```python
from build123d import *

# Parameters (mm, degrees)
F0_R     = 1.5875
F0_W     = 3.175
F0_H     = 10.004552
F1_DEPTH = 3.175


# Not quite as in the source:
# - a length typed as a fraction of an inch, garbled in the dataset ("3 / 203.2 mm" for 3/8 in), is restored
# - a feature names something its author has since deleted; it is built from what else it names


with BuildPart() as f1:
    # F0 (on Top) → F1 (new body)
    with BuildSketch(Plane.XY):
        with BuildLine():
            Line((-226.9615088272, -74.910188), (-188.8615088272, -74.910188))
            ThreePointArc((-188.8615088272, -74.910188), (-180.8069453098, -55.4647515174), (-161.3615088272, -47.410188))
            ThreePointArc((-161.3615088272, -47.410188), (-141.9160723446, -55.4647515174), (-133.8615088272, -74.910188))
            Line((-133.8615088272, -74.910188), (-95.7615088272, -74.910188))
            Line((-95.7615088272, -74.910188), (-95.7615088272, 102.889812))
            Line((-95.7615088272, 102.889812), (-226.9615088272, 102.889812))
            Line((-226.9615088272, 102.889812), (-226.9615088272, -74.910188))
        make_face()
        Polygon((-221.8815088272, 50.02276), (-221.8815088272, 60.027312), (-218.7065088272, 60.027312), (-218.7065088272, 50.02276), (-218.7065088272, 40.018208), (-218.7065088272, 30.013656), (-218.7065088272, 20.009104), (-218.7065088272, 10.004552), (-218.7065088272, 0), (-218.7065088272, -10.004552), (-218.7065088272, -20.009104), (-218.7065088272, -30.013656), (-218.7065088272, -40.018208), (-218.7065088272, -50.02276), (-221.8815088272, -50.02276), (-221.8815088272, -40.018208), (-221.8815088272, -30.013656), (-221.8815088272, -20.009104), (-221.8815088272, -10.004552), (-221.8815088272, 0), (-221.8815088272, 10.004552), (-221.8815088272, 20.009104), (-221.8815088272, 30.013656), (-221.8815088272, 40.018208), align=None, mode=Mode.SUBTRACT)
        Polygon((-199.6565088272, 60.027312), (-196.4815088272, 60.027312), (-196.4815088272, 50.02276), (-196.4815088272, 40.018208), (-196.4815088272, 30.013656), (-196.4815088272, 20.009104), (-196.4815088272, 10.004552), (-196.4815088272, 0), (-196.4815088272, -10.004552), (-196.4815088272, -20.009104), (-196.4815088272, -30.013656), (-196.4815088272, -40.018208), (-196.4815088272, -50.02276), (-199.6565088272, -50.02276), (-199.6565088272, -40.018208), (-199.6565088272, -30.013656), (-199.6565088272, -20.009104), (-199.6565088272, -10.004552), (-199.6565088272, 0), (-199.6565088272, 10.004552), (-199.6565088272, 20.009104), (-199.6565088272, 30.013656), (-199.6565088272, 40.018208), (-199.6565088272, 50.02276), align=None, mode=Mode.SUBTRACT)
        with Locations((-186.3334280729, -16.5444072336)):
            Circle(F0_R, mode=Mode.SUBTRACT)
        Polygon((-126.2415088272, 60.027312), (-123.0665088272, 60.027312), (-123.0665088272, 50.02276), (-123.0665088272, 40.018208), (-123.0665088272, 30.013656), (-123.0665088272, 20.009104), (-123.0665088272, 10.004552), (-123.0665088272, 0), (-123.0665088272, -10.004552), (-123.0665088272, -20.009104), (-123.0665088272, -30.013656), (-123.0665088272, -40.018208), (-123.0665088272, -50.02276), (-126.2415088272, -50.02276), (-126.2415088272, -40.018208), (-126.2415088272, -30.013656), (-126.2415088272, -20.009104), (-126.2415088272, -10.004552), (-126.2415088272, 0), (-126.2415088272, 10.004552), (-126.2415088272, 20.009104), (-126.2415088272, 30.013656), (-126.2415088272, 40.018208), (-126.2415088272, 50.02276), align=None, mode=Mode.SUBTRACT)
        Polygon((-104.0165088272, 50.02276), (-104.0165088272, 60.027312), (-100.8415088272, 60.027312), (-100.8415088272, 50.02276), (-100.8415088272, 40.018208), (-100.8415088272, 30.013656), (-100.8415088272, 20.009104), (-100.8415088272, 10.004552), (-100.8415088272, 0), (-100.8415088272, -10.004552), (-100.8415088272, -20.009104), (-100.8415088272, -30.013656), (-100.8415088272, -40.018208), (-100.8415088272, -50.02276), (-104.0165088272, -50.02276), (-104.0165088272, -40.018208), (-104.0165088272, -30.013656), (-104.0165088272, -20.009104), (-104.0165088272, -10.004552), (-104.0165088272, 0), (-104.0165088272, 10.004552), (-104.0165088272, 20.009104), (-104.0165088272, 30.013656), (-104.0165088272, 40.018208), align=None, mode=Mode.SUBTRACT)
        with BuildLine():
            ThreePointArc((-158.8215088272, 92.729812), (-159.565457603, 90.9337607758), (-161.3615088272, 90.189812))
            ThreePointArc((-161.3615088272, 90.189812), (-163.1575600514, 94.5258632242), (-158.8215088272, 92.729812))
        make_face(mode=Mode.SUBTRACT)
        with Locations((-143.4709280729, 34.2555927664)):
            Circle(F0_R, mode=Mode.SUBTRACT)
        with Locations((-198.0690088272, -45.020484)):
            Rectangle(F0_W, F0_H)
        with Locations((-198.0690088272, -25.01138)):
            Rectangle(F0_W, F0_H)
        with Locations((-198.0690088272, -5.002276)):
            Rectangle(F0_W, F0_H)
        with Locations((-198.0690088272, 15.006828)):
            Rectangle(F0_W, F0_H)
        with Locations((-198.0690088272, 35.015932)):
            Rectangle(F0_W, F0_H)
        with Locations((-198.0690088272, 55.025036)):
            Rectangle(F0_W, F0_H)
        with Locations((-220.2940088272, -35.015932)):
            Rectangle(F0_W, F0_H)
        with Locations((-220.2940088272, -15.006828)):
            Rectangle(F0_W, F0_H)
        with Locations((-220.2940088272, 5.002276)):
            Rectangle(F0_W, F0_H)
        with Locations((-220.2940088272, 25.01138)):
            Rectangle(F0_W, F0_H)
        with Locations((-220.2940088272, 45.020484)):
            Rectangle(F0_W, F0_H)
        with Locations((-102.4290088272, 45.020484)):
            Rectangle(F0_W, F0_H)
        with Locations((-102.4290088272, 25.01138)):
            Rectangle(F0_W, F0_H)
        with Locations((-102.4290088272, 5.002276)):
            Rectangle(F0_W, F0_H)
        with Locations((-102.4290088272, -15.006828)):
            Rectangle(F0_W, F0_H)
        with Locations((-102.4290088272, -35.015932)):
            Rectangle(F0_W, F0_H)
        with Locations((-124.6540088272, 55.025036)):
            Rectangle(F0_W, F0_H)
        with Locations((-124.6540088272, 35.015932)):
            Rectangle(F0_W, F0_H)
        with Locations((-124.6540088272, 15.006828)):
            Rectangle(F0_W, F0_H)
        with Locations((-124.6540088272, -5.002276)):
            Rectangle(F0_W, F0_H)
        with Locations((-124.6540088272, -25.01138)):
            Rectangle(F0_W, F0_H)
        with Locations((-124.6540088272, -45.020484)):
            Rectangle(F0_W, F0_H)
    extrude(amount=F1_DEPTH)


solid = f1.part
```
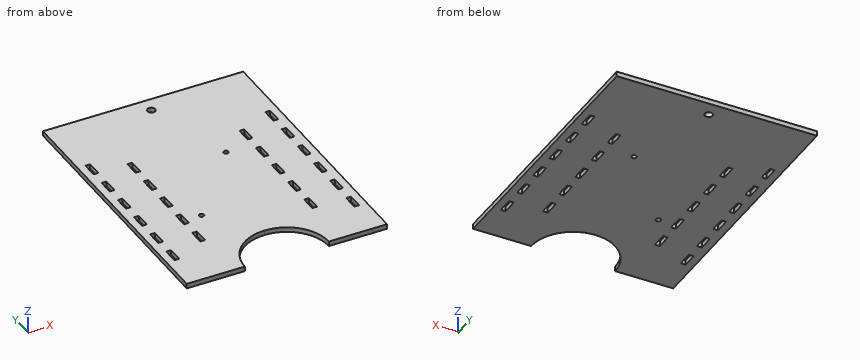
Can you work these out from the model? Positions are in its coordinate system, mm. Coordinates: 2 decimals unless noted, no trailing zeros. Write each loop counter-clockwise with the first axis right and the second up, starting at its lowest first coordinate (ties: lowest second). Pieces come first, ordered by that corner, then holes. Notation, with made-up numbers: (-9, -4.5) - (45, -4.5) arc R7 cw to (45, 8.5) - close; hole circle Ø6 at (41.5, 17). An arc over 180 degrees is marked (long way). Return JSON: item names as keys, results as strings.
Q1. Please list where these lines run through material, in increasing order: L1, parallel to X at y = 57, z = 1.55; L2, parallel to X at y = -17, z = 1.75; L3, parallel to X at y = -51.5, z = 0.6. Write a range as from..to.
Computed values:
{"L1": "x = -226.96..-221.88, -218.71..-104.02, -100.84..-95.76", "L2": "x = -226.96..-199.66, -196.48..-187.85, -184.81..-126.24, -123.07..-95.76", "L3": "x = -226.96..-175.79, -146.93..-95.76"}
Q2. If we section it at B-B (x = -155): Please give me the cut outline in (y, z) (3 decimals), then the cut area to 3 significant figures.
Computed values:
{"outline": "(-48.156, 0) - (102.89, 0) - (102.89, 3.175) - (-48.156, 3.175) - close", "area": "480 mm2"}
Q3. If we section it at C-C (z = 0.75): Count the separate pieces of the cut face and the enclosed holes in it, then the cut area to 3 significant figures.
Computed values:
{"separate pieces": "1", "enclosed holes": "25", "area": "21,400 mm2"}
Q4. If we section it at A-A (y = 2): Please give me the cut outline in (x, z) (1 decimal).
Computed values:
{"outline": "(-227, 0) - (-199.7, 0) - (-199.7, 3.2) - (-227, 3.2) - close; (-196.5, 0) - (-126.2, 0) - (-126.2, 3.2) - (-196.5, 3.2) - close; (-123.1, 0) - (-95.8, 0) - (-95.8, 3.2) - (-123.1, 3.2) - close"}
Q5. I'm going to push a flat-ended pin straight in: pin 1 Ø10 at (x, y) = (-113.5, -6) entering from -Z. Where does the tip first touch, or does it pass through?
Computed values:
{"pin 1": "stops at z = 0"}
